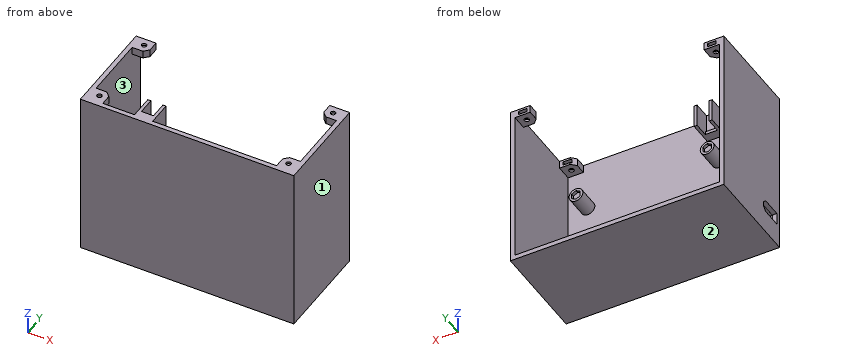
```python
from build123d import *

# Parameters (mm, degrees)
SKETCH_2_W          = 140
SKETCH_2_H          = 65
EXTRUDE_1_DEPTH     = 110
SKETCH_3_W          = 134
SKETCH_3_H          = 107
CUT_EXTRUDE_1_DEPTH = 62
SKETCH_4_W          = 10
SKETCH_4_H          = 10
SKETCH_4_R          = 1.6
EXTRUDE_2_DEPTH     = 5
SKETCH_5_W          = 10
SKETCH_5_H          = 10
SKETCH_5_R          = 1.6
EXTRUDE_3_DEPTH     = 5
SKETCH_6_W          = 5.5
SKETCH_6_H          = 2.3
CUT_EXTRUDE_2_DEPTH = 8
SKETCH_8_W          = 5.5
SKETCH_8_H          = 2.3
CUT_EXTRUDE_3_DEPTH = 8
CHAMFER_1_SIZE      = 3
SKETCH_9_R          = 4.5
EXTRUDE_4_DEPTH     = 14
CUT_EXTRUDE_4_DEPTH = 2
CUT_EXTRUDE_5_REACH = 182.987
EXTRUDE_5_DEPTH     = 11
SKETCH_16_W         = 5.817441426
SKETCH_16_H         = 7.857396667
CUT_EXTRUDE_6_DEPTH = 9
EXTRUDE_6_DEPTH     = 15.5
SKETCH_18_W         = 7.9
SKETCH_18_H         = 11.370001712
CUT_EXTRUDE_7_DEPTH = 9.5
SKETCH_19_W         = 7.9
SKETCH_19_H         = 13
EXTRUDE_7_DEPTH     = 4.5


with BuildPart() as part:
    # Эскиз2 → Бобышка-Вытянуть1 (new body)
    with BuildSketch(Plane.XY):
        Rectangle(SKETCH_2_W, SKETCH_2_H)
    extrude(amount=EXTRUDE_1_DEPTH)

    # Эскиз3 → Вырез-Вытянуть1 (cut)
    with BuildSketch(Plane(origin=(0, 32.5, 0), x_dir=(1, 0, 0), z_dir=(0, 1, 0))):
        with Locations((0, -56.5)):
            Rectangle(SKETCH_3_W, SKETCH_3_H)
    extrude(amount=-CUT_EXTRUDE_1_DEPTH, mode=Mode.SUBTRACT)

    # Эскиз4 → Бобышка-Вытянуть2 (add)
    # profile 1 of 2: a face of its own
    with BuildSketch(Plane.XY.offset(110)):
        with Locations((62, -24.5)):
            Rectangle(SKETCH_4_W, SKETCH_4_H)
        with Locations((62, -24.5)):
            Circle(SKETCH_4_R, mode=Mode.SUBTRACT)
    # profile 2 of 2: a face of its own
    with BuildSketch(Plane.XY.offset(110)):
        with Locations((-62, -24.5)):
            Rectangle(SKETCH_4_W, SKETCH_4_H)
        with Locations((-62, -24.5)):
            Circle(SKETCH_4_R, mode=Mode.SUBTRACT)
    extrude(amount=-EXTRUDE_2_DEPTH)

    # Эскиз5 → Бобышка-Вытянуть3 (add)
    # profile 1 of 2: a face of its own
    with BuildSketch(Plane.XY.offset(110)):
        with Locations((62, 27.5)):
            Rectangle(SKETCH_5_W, SKETCH_5_H)
        with Locations((62, 27.5)):
            Circle(SKETCH_5_R, mode=Mode.SUBTRACT)
    # profile 2 of 2: a face of its own
    with BuildSketch(Plane.XY.offset(110)):
        with Locations((-62, 27.5)):
            Rectangle(SKETCH_5_W, SKETCH_5_H)
        with Locations((-62, 27.5)):
            Circle(SKETCH_5_R, mode=Mode.SUBTRACT)
    extrude(amount=-EXTRUDE_3_DEPTH)

    # Эскиз6 → Вырез-Вытянуть2 (cut)
    with BuildSketch(Plane(origin=(0, 32.5, 0), x_dir=(1, 0, 0), z_dir=(0, 1, 0))):
        with Locations((-62, -107.5)):
            Rectangle(SKETCH_6_W, SKETCH_6_H)
        with Locations((62, -107.5)):
            Rectangle(SKETCH_6_W, SKETCH_6_H)
    extrude(amount=-CUT_EXTRUDE_2_DEPTH, mode=Mode.SUBTRACT)

    # Эскиз8 → Вырез-Вытянуть3 (cut)
    with BuildSketch(Plane(origin=(0, -19.5, 0), x_dir=(1, 0, 0), z_dir=(0, 1, 0))):
        with Locations((62, -107.5)):
            Rectangle(SKETCH_8_W, SKETCH_8_H)
        with Locations((-62, -107.5)):
            Rectangle(SKETCH_8_W, SKETCH_8_H)
    extrude(amount=-CUT_EXTRUDE_3_DEPTH, mode=Mode.SUBTRACT)

    # Фаска1
    # the kernel refuses this chamfer: 3 mm, written as the material it takes off along each edge
    with BuildSketch(Plane(origin=(57, 22.5, 117.715048964), x_dir=(-0.027495876610586768, 0.9996219169112968, 0), z_dir=(0, 0, -1))) as chamfer_1_piece_1:
        Polygon((CHAMFER_1_SIZE * 0.999621916911, CHAMFER_1_SIZE * 0.0274958766106), (-CHAMFER_1_SIZE * 0.0274958766106, CHAMFER_1_SIZE * 0.999621916911), (0, 0), align=None)
    extrude(amount=20.430097928, mode=Mode.SUBTRACT)
    with BuildSketch(Plane(origin=(57, -19.5, 117.715048964), x_dir=(-0.027495876610586768, -0.9996219169112968, 0), z_dir=(0, 0, -1)), Plane(origin=(-57, 22.5, 117.715048964), x_dir=(0.027495876610586733, 0.9996219169112968, 0), z_dir=(0, 0, -1)), Plane(origin=(-57, -19.5, 117.715048964), x_dir=(-0.9996219169112965, 0.02749587661058676, 0), z_dir=(0, 0, -1))) as chamfer_1_piece_2:
        Polygon((CHAMFER_1_SIZE * 0.999621916911, -CHAMFER_1_SIZE * 0.0274958766106), (-CHAMFER_1_SIZE * 0.0274958766106, -CHAMFER_1_SIZE * 0.999621916911), (0, 0), align=None)
    extrude(amount=20.430097928, mode=Mode.SUBTRACT)

    # Эскиз9 → Бобышка-Вытянуть4 (add)
    with BuildSketch(Plane(origin=(0, -29.5, 0), x_dir=(1, 0, 0), z_dir=(0, 1, 0))):
        with Locations(Location((54, -13, 0), (0, 0, 270))):
            Circle(SKETCH_9_R)
        with Locations(Location((-32, -13, 0), (0, 0, 270))):
            Circle(SKETCH_9_R)
        with Locations(Location((-32, -77, 0), (0, 0, 270))):
            Circle(SKETCH_9_R)
        with Locations(Location((54, -77, 0), (0, 0, 270))):
            Circle(SKETCH_9_R)
    extrude(amount=EXTRUDE_4_DEPTH)

    # Эскиз12 → Вырез-Вытянуть4 (cut)
    with BuildSketch(Plane(origin=(0, -15.5, 0), x_dir=(1, 0, 0), z_dir=(0, 1, 0))):
        Polygon((54, -9.766838493), (51.2, -11.383419246), (51.2, -14.616580754), (54, -16.233161507), (56.8, -14.616580754), (56.8, -11.383419246), align=None)
        Polygon((-32, -9.766838493), (-34.8, -11.383419246), (-34.8, -14.616580754), (-32, -16.233161507), (-29.2, -14.616580754), (-29.2, -11.383419246), align=None)
        Polygon((54, -73.766838493), (51.2, -75.383419246), (51.2, -78.616580754), (54, -80.233161507), (56.8, -78.616580754), (56.8, -75.383419246), align=None)
        Polygon((-32, -73.766838493), (-34.8, -75.383419246), (-34.8, -78.616580754), (-32, -80.233161507), (-29.2, -78.616580754), (-29.2, -75.383419246), align=None)
    extrude(amount=-CUT_EXTRUDE_4_DEPTH, mode=Mode.SUBTRACT)

    # Эскиз13 → Вырез-Вытянуть5 (cut, up to next)
    with BuildSketch(Plane.ZY.offset(70), mode=Mode.PRIVATE) as cut_extrude_5_sk1:
        Polygon((15, -29.3), (22.9, -29.3), (22.9, -16.2), (20.405788704, -13.7), (17.494211296, -13.7), (15, -16.2), align=None)
    cut_extrude_5_tool1 = extrude(cut_extrude_5_sk1.sketch, amount=-CUT_EXTRUDE_5_REACH, mode=Mode.PRIVATE) & part.part
    add(cut_extrude_5_tool1.solids().sort_by_distance((-70, -21.871275, 18.95))[0], mode=Mode.SUBTRACT)

    # Эскиз15 → Бобышка-Вытянуть5 (add)
    with BuildSketch(Plane(origin=(0, -29.5, 0), x_dir=(1, 0, 0), z_dir=(0, 1, 0))):
        Polygon((-67, -24.878202282), (-52, -24.878202282), (-52, -12.978202282), (-67, -12.978202282), (-67, -14.978202282), (-54, -14.978202282), (-54, -22.878202282), (-67, -22.878202282), align=None)
    extrude(amount=EXTRUDE_5_DEPTH)

    # Эскиз16 → Вырез-Вытянуть6 (cut)
    with BuildSketch(Plane(origin=(0, -18.5, 0), x_dir=(1, 0, 0), z_dir=(0, 1, 0))):
        with Locations((-52, -18.928202283)):
            Rectangle(SKETCH_16_W, SKETCH_16_H)
    extrude(amount=-CUT_EXTRUDE_6_DEPTH, mode=Mode.SUBTRACT)

    # Эскиз17 → Бобышка-Вытянуть6 (add)
    with BuildSketch(Plane(origin=(0, -29.5, 0), x_dir=(1, 0, 0), z_dir=(0, 1, 0))):
        Polygon((-36.2, -110), (-36.2, -95), (-24.3, -95), (-24.3, -110), (-26.3, -110), (-26.3, -97), (-34.2, -97), (-34.2, -110), align=None)
    extrude(amount=EXTRUDE_6_DEPTH)

    # Эскиз18 → Вырез-Вытянуть7 (cut)
    with BuildSketch(Plane(origin=(0, -14, 0), x_dir=(1, 0, 0), z_dir=(0, 1, 0))):
        with Locations((-30.25, -95)):
            Rectangle(SKETCH_18_W, SKETCH_18_H)
    extrude(amount=-CUT_EXTRUDE_7_DEPTH, mode=Mode.SUBTRACT)

    # Эскиз19 → Бобышка-Вытянуть7 (add)
    with BuildSketch(Plane(origin=(0, -29.5, 0), x_dir=(1, 0, 0), z_dir=(0, 1, 0))):
        with Locations((-30.25, -103.5)):
            Rectangle(SKETCH_19_W, SKETCH_19_H)
    extrude(amount=EXTRUDE_7_DEPTH)


solid = part.part
```
The model under review builds one solid part; all positions refer to its coordinate system, in mm. Face numbers are marked on the shaded views. Round coordinates to 2 decimals unless told otherwise and drop trailing zeros. Order: outer loops, then holes, each group sorted by start corner. A loop starts at its lowest first (then second) coordinate and runs counter-clockwise, first axis right, second up.
(1) Take a section at C-C, the plane y = 27.5. Count the separate pieces of the cut face and the enclosed holes in it, plus the area to 3 significant figures.
Working result:
separate pieces: 3
enclosed holes: 0
area: 1,120 mm2
(2) Take a section at A-A, the plane z = 52. State the section outline as (x, y) points.
Working result:
outline: (-70, -32.5) - (70, -32.5) - (70, 32.5) - (67, 32.5) - (67, -29.5) - (-67, -29.5) - (-67, 32.5) - (-70, 32.5) - close
(3) Wall thickness on L1, parallel to Y at x = -62, z = 106; L2, parallel to X at y = -21.5, z = 28; L3, parallel to Z at x = 60.5, y = -29: over which ranges is each line inside the solid? List them lowest first.
Working result:
L1: y = -32.5 to -26.1, -22.9 to -19.5, 22.5 to 25.9, 29.1 to 32.5
L2: x = -70 to -67, 67 to 70
L3: z = 0 to 3, 105 to 110
(4) For P1, Ø6, axis at x = -6.5, z = 54, coming from the +Y side; P2, Ø3.5, axis at x = -62, y = 27.5, coming from the +Z side; P3, Ø1.7, axis at x = -32.5, z = 76.5, coming from the +Y side; P4, Ø5, axis at x = -28.5, y = 24.5, coming from the +Z side, all flat-tipped, find the tip position at first contact; note any pin that passes through.
Working result:
P1: stops at y = -29.5
P2: stops at z = 110
P3: stops at y = -17.5
P4: stops at z = 3
(5) Take a section at B-B, the plane x = 44. State the section outline as (y, z) points, plus the area to 3 significant figures.
Working result:
outline: (-32.5, 0) - (32.5, 0) - (32.5, 3) - (-29.5, 3) - (-29.5, 110) - (-32.5, 110) - close
area: 516 mm2
(6) Mouldability with a two-part tool opening along Z and no side actions: class the marked faces 1, 2 and 3 as released by +Z, released by -Z, zero draft, split by the parting line, or undercut.
Working result:
face 1: zero draft
face 2: released by -Z
face 3: undercut
